```python
from build123d import *
from OCP.BRepFilletAPI import BRepFilletAPI_MakeChamfer

# Parameters (mm, degrees)
SKETCH_1_W                  = 85
SKETCH_1_H                  = 54
EXTRUDE_576_DEPTH           = 7.5
FILLET_627_R                = 3
CUT_EXTRUDE_1389_DEPTH      = 5.5
FILLET_1467_R               = 1
EXTRUDE_2395_DEPTH          = 2
CHAMFER_2448_SIZE           = 1
CHAMFER_2448_SIZE2          = 0.176326981
SKETCH_16_R                 = 2.5
CUT_EXTRUDE_2683_DEPTH      = 5
SKETCH_19_W                 = 7.62
SKETCH_19_H                 = 5.08
CUT_EXTRUDE_3124_DEPTH      = 10
SKETCH_21_W                 = 11.1
SKETCH_21_H                 = 1.1
CUT_EXTRUDE_2_DEPTH         = 10
SKETCH_22_W                 = 2.8
SKETCH_22_H                 = 1.2
CUT_EXTRUDE_3_DEPTH         = 10
CUT_EXTRUDE_5_DEPTH         = 10
SKETCH_30_W                 = 11.1
SKETCH_30_H                 = 0.725
SKETCH_30_W_2               = 2.8
SKETCH_30_H_2               = 1.3
CUT_EXTRUDE_6_DEPTH         = 1
EXTRUDE_2_DEPTH             = 1
EXTRUDE_3_DEPTH             = 1
CUT_EXTRUDE_START           = -1
SKETCH_31_W                 = 7.6
SKETCH_31_H                 = 0.55
SKETCH_31_W_2               = 5
SKETCH_31_H_2               = 2
CUT_EXTRUDE_7_DEPTH         = 1
SKETCH_32_W                 = 2.8
SKETCH_32_H                 = 1.2
CUT_EXTRUDE_8_DEPTH         = 10
SKETCH_33_W                 = 2.8
SKETCH_33_H                 = 1.3
CUT_EXTRUDE_9_DEPTH         = 2
SKETCH_34_R                 = 3
SKETCH_34_R_2               = 1.5
EXTRUDE_4_DEPTH             = 3.4
PATTERN_LINEAR_1_COUNT      = 2
PATTERN_LINEAR_1_PITCH      = 74
PATTERN_LINEAR_1_COUNT_DIR2 = 2
PATTERN_LINEAR_1_PITCH_DIR2 = 43


with BuildPart() as part:
    # 草图1 → Extrude 576 (new body)
    with BuildSketch(Plane(origin=(0, 0, 0), x_dir=(1, 0, 0), z_dir=(0, 1, 0))):
        Rectangle(SKETCH_1_W, SKETCH_1_H)
    extrude(amount=EXTRUDE_576_DEPTH)

    # Fillet 627
    fillet_627_edges = [part.edges().sort_by_distance(p)[0] for p in [
        (0, 0, 27),
        (-42.5, 0, 0),
        (0, 0, -27),
        (42.5, 0, 0),
        (42.5, 3.75, 27),
        (-42.5, 3.75, 27),
        (-42.5, 3.75, -27),
        (42.5, 3.75, -27),
    ]]
    fillet(fillet_627_edges, radius=FILLET_627_R)

    # 草图14 → Cut-Extrude 1389 (cut)
    with BuildSketch(Plane(origin=(0, 7.5, 0), x_dir=(1, 0, 0), z_dir=(0, 1, 0))):
        with BuildLine():
            Line((-39.5, -25), (39.5, -25))
            ThreePointArc((39.5, -25), (40.207106781, -24.707106781), (40.5, -24))
            Line((40.5, -24), (40.5, 24))
            ThreePointArc((40.5, 24), (40.207106781, 24.707106781), (39.5, 25))
            Line((39.5, 25), (-39.5, 25))
            ThreePointArc((-39.5, 25), (-40.207106781, 24.707106781), (-40.5, 24))
            Line((-40.5, 24), (-40.5, -24))
            ThreePointArc((-40.5, -24), (-40.207106781, -24.707106781), (-39.5, -25))
        make_face()
    extrude(amount=-CUT_EXTRUDE_1389_DEPTH, mode=Mode.SUBTRACT)

    # Fillet 1467
    fillet_1467_edges = [part.edges().sort_by_distance(p)[0] for p in [
        (40.207106781, 2, 24.707106781),
        (0, 2, 25),
        (-40.207106781, 2, 24.707106781),
        (-40.5, 2, 0),
        (-40.207106781, 2, -24.707106781),
        (0, 2, -25),
        (40.207106781, 2, -24.707106781),
        (40.5, 2, 0),
    ]]
    fillet(fillet_1467_edges, radius=FILLET_1467_R)

    # 草图15 → Extrude 2395 (add)
    with BuildSketch(Plane(origin=(0, 7.5, 0), x_dir=(1, 0, 0), z_dir=(0, 1, 0))):
        with BuildLine():
            Line((-39.5, -26), (39.5, -26))
            ThreePointArc((39.5, -26), (40.914213562, -25.414213562), (41.5, -24))
            Line((41.5, -24), (41.5, 24))
            ThreePointArc((41.5, 24), (40.914213562, 25.414213562), (39.5, 26))
            Line((39.5, 26), (-39.5, 26))
            ThreePointArc((-39.5, 26), (-40.914213562, 25.414213562), (-41.5, 24))
            Line((-41.5, 24), (-41.5, -24))
            ThreePointArc((-41.5, -24), (-40.914213562, -25.414213562), (-39.5, -26))
        make_face()
        with BuildLine():
            Line((-39.5, -25), (39.5, -25))
            ThreePointArc((39.5, -25), (40.207106781, -24.707106781), (40.5, -24))
            Line((40.5, -24), (40.5, 24))
            ThreePointArc((40.5, 24), (40.207106781, 24.707106781), (39.5, 25))
            Line((39.5, 25), (-39.5, 25))
            ThreePointArc((-39.5, 25), (-40.207106781, 24.707106781), (-40.5, 24))
            Line((-40.5, 24), (-40.5, -24))
            ThreePointArc((-40.5, -24), (-40.207106781, -24.707106781), (-39.5, -25))
        make_face(mode=Mode.SUBTRACT)
    extrude(amount=EXTRUDE_2395_DEPTH)

    # Chamfer 2448: one chamfer whose edges measure the first distance from different faces: ONE call of the kernel's chamfer builder (chamfer() names one face for all edges)
    chamfer_2448_edges_1 = [part.edges().sort_by_distance(p)[0] for p in [
        (-40.914213562, 9.5, 25.414213562),
    ]]
    chamfer_2448_side_1 = [part.faces().sort_by_distance(p)[0] for p in [
        (-40.914213562, 8.5, 25.414213562),
    ]]
    chamfer_2448_edges_2 = [part.edges().sort_by_distance(p)[0] for p in [
        (0, 9.5, 26),
    ]]
    chamfer_2448_side_2 = [part.faces().sort_by_distance(p)[0] for p in [
        (0, 8.5, 26),
    ]]
    chamfer_2448_edges_3 = [part.edges().sort_by_distance(p)[0] for p in [
        (40.914213562, 9.5, 25.414213562),
    ]]
    chamfer_2448_side_3 = [part.faces().sort_by_distance(p)[0] for p in [
        (40.914213562, 8.5, 25.414213562),
    ]]
    chamfer_2448_edges_4 = [part.edges().sort_by_distance(p)[0] for p in [
        (41.5, 9.5, 0),
    ]]
    chamfer_2448_side_4 = [part.faces().sort_by_distance(p)[0] for p in [
        (41.5, 8.5, 0),
    ]]
    chamfer_2448_edges_5 = [part.edges().sort_by_distance(p)[0] for p in [
        (40.914213562, 9.5, -25.414213562),
    ]]
    chamfer_2448_side_5 = [part.faces().sort_by_distance(p)[0] for p in [
        (40.914213562, 8.5, -25.414213562),
    ]]
    chamfer_2448_edges_6 = [part.edges().sort_by_distance(p)[0] for p in [
        (0, 9.5, -26),
    ]]
    chamfer_2448_side_6 = [part.faces().sort_by_distance(p)[0] for p in [
        (0, 8.5, -26),
    ]]
    chamfer_2448_edges_7 = [part.edges().sort_by_distance(p)[0] for p in [
        (-40.914213562, 9.5, -25.414213562),
    ]]
    chamfer_2448_side_7 = [part.faces().sort_by_distance(p)[0] for p in [
        (-40.914213562, 8.5, -25.414213562),
    ]]
    chamfer_2448_edges_8 = [part.edges().sort_by_distance(p)[0] for p in [
        (-41.5, 9.5, 0),
    ]]
    chamfer_2448_side_8 = [part.faces().sort_by_distance(p)[0] for p in [
        (-41.5, 8.5, 0),
    ]]
    chamfer_2448 = BRepFilletAPI_MakeChamfer(part.part.solid().wrapped)
    for e in chamfer_2448_edges_1:
        chamfer_2448.Add(CHAMFER_2448_SIZE, CHAMFER_2448_SIZE2, e.wrapped, chamfer_2448_side_1[0].wrapped)  # the first distance lies on this face
    for e in chamfer_2448_edges_2:
        chamfer_2448.Add(CHAMFER_2448_SIZE, CHAMFER_2448_SIZE2, e.wrapped, chamfer_2448_side_2[0].wrapped)  # the first distance lies on this face
    for e in chamfer_2448_edges_3:
        chamfer_2448.Add(CHAMFER_2448_SIZE, CHAMFER_2448_SIZE2, e.wrapped, chamfer_2448_side_3[0].wrapped)  # the first distance lies on this face
    for e in chamfer_2448_edges_4:
        chamfer_2448.Add(CHAMFER_2448_SIZE, CHAMFER_2448_SIZE2, e.wrapped, chamfer_2448_side_4[0].wrapped)  # the first distance lies on this face
    for e in chamfer_2448_edges_5:
        chamfer_2448.Add(CHAMFER_2448_SIZE, CHAMFER_2448_SIZE2, e.wrapped, chamfer_2448_side_5[0].wrapped)  # the first distance lies on this face
    for e in chamfer_2448_edges_6:
        chamfer_2448.Add(CHAMFER_2448_SIZE, CHAMFER_2448_SIZE2, e.wrapped, chamfer_2448_side_6[0].wrapped)  # the first distance lies on this face
    for e in chamfer_2448_edges_7:
        chamfer_2448.Add(CHAMFER_2448_SIZE, CHAMFER_2448_SIZE2, e.wrapped, chamfer_2448_side_7[0].wrapped)  # the first distance lies on this face
    for e in chamfer_2448_edges_8:
        chamfer_2448.Add(CHAMFER_2448_SIZE, CHAMFER_2448_SIZE2, e.wrapped, chamfer_2448_side_8[0].wrapped)  # the first distance lies on this face
    add(Compound.cast(chamfer_2448.Shape()), mode=Mode.REPLACE)

    # 草图16 → Cut-Extrude 2683 (cut)
    with BuildSketch(Plane(origin=(42.5, 0, 0), x_dir=(0, 0, -1), z_dir=(1, 0, 0))):
        with Locations((13, 7.5)):
            Circle(SKETCH_16_R)
    extrude(amount=-CUT_EXTRUDE_2683_DEPTH, mode=Mode.SUBTRACT)

    # 草图19 → Cut-Extrude 3124 (cut)
    with BuildSketch(Plane(origin=(42.5, 0, 0), x_dir=(0, 0, -1), z_dir=(1, 0, 0))):
        with Locations((-14.978380782, 7.5)):
            Rectangle(SKETCH_19_W, SKETCH_19_H)
    extrude(amount=-CUT_EXTRUDE_3124_DEPTH, mode=Mode.SUBTRACT)

    # 草图21 → 切除-拉伸2 (cut)
    with BuildSketch(Plane.ZY.offset(42.5)):
        with Locations((0, 8.225)):
            Rectangle(SKETCH_21_W, SKETCH_21_H)
    extrude(amount=-CUT_EXTRUDE_2_DEPTH, mode=Mode.SUBTRACT)

    # 草图22 → 切除-拉伸3 (cut)
    with BuildSketch(Plane.ZY.offset(42.5)):
        with Locations((15.5, 7.6)):
            Rectangle(SKETCH_22_W, SKETCH_22_H)
    extrude(amount=-CUT_EXTRUDE_3_DEPTH, mode=Mode.SUBTRACT)

    # 草图25 → 切除-拉伸5 (cut)
    with BuildSketch(Plane(origin=(42.5, 0, 0), x_dir=(0, 0, -1), z_dir=(1, 0, 0))):
        with BuildLine():
            Line((3.8, 8.257106781), (3.8, 8.95))
            ThreePointArc((3.8, 8.95), (3.653553391, 9.303553391), (3.3, 9.45))
            Line((3.3, 9.45), (-3.3, 9.45))
            ThreePointArc((-3.3, 9.45), (-3.653553391, 9.303553391), (-3.8, 8.95))
            Line((-3.8, 8.95), (-3.8, 8.257106781))
            ThreePointArc((-3.8, 8.257106781), (-3.761939766, 8.065765065), (-3.653553391, 7.903553391))
            Line((-3.653553391, 7.903553391), (-2.746446609, 6.996446609))
            ThreePointArc((-2.746446609, 6.996446609), (-2.584234935, 6.888060234), (-2.392893219, 6.85))
            Line((-2.392893219, 6.85), (2.392893219, 6.85))
            ThreePointArc((2.392893219, 6.85), (2.584234935, 6.888060234), (2.746446609, 6.996446609))
            Line((2.746446609, 6.996446609), (3.653553391, 7.903553391))
            ThreePointArc((3.653553391, 7.903553391), (3.761939766, 8.065765065), (3.8, 8.257106781))
        make_face()
    extrude(amount=-CUT_EXTRUDE_5_DEPTH, mode=Mode.SUBTRACT)

    # 草图30 → 切除-拉伸6 (cut)
    with BuildSketch(Plane.ZY.offset(41.5)):
        with Locations((0, 9.1375)):
            Rectangle(SKETCH_30_W, SKETCH_30_H)
        with Locations((15.5, 8.85)):
            Rectangle(SKETCH_30_W_2, SKETCH_30_H_2)
    extrude(amount=-CUT_EXTRUDE_6_DEPTH, mode=Mode.SUBTRACT)

    # 草图28 → 凸台-拉伸2 (add)
    with BuildSketch(Plane(origin=(41.5, 0, 0), x_dir=(0, 0, -1), z_dir=(1, 0, 0))):
        with BuildLine():
            Line((3.653553391, 7.903553391), (3.25, 7.5))
            Line((3.25, 7.5), (4.237115804, 7.5))
            Line((4.237115804, 7.5), (3.8, 8.257106781))
            ThreePointArc((3.8, 8.257106781), (3.761939766, 8.065765065), (3.653553391, 7.903553391))
        make_face()
        with BuildLine():
            Line((-3.25, 7.5), (-3.653553391, 7.903553391))
            ThreePointArc((-3.653553391, 7.903553391), (-3.761939766, 8.065765065), (-3.8, 8.257106781))
            Line((-3.8, 8.257106781), (-4.237115804, 7.5))
            Line((-4.237115804, 7.5), (-3.25, 7.5))
        make_face()
    extrude(amount=EXTRUDE_2_DEPTH)

    # 草图29 → 凸台-拉伸3 (add)
    with BuildSketch(Plane.ZY.offset(41.5)):
        Polygon((-5.55, 7.675), (-5.651036297, 7.5), (5.651036297, 7.5), (5.55, 7.675), align=None)
    extrude(amount=EXTRUDE_3_DEPTH)

    # 草图31 → 切除-拉伸7 (cut)
    with BuildSketch(Plane(origin=(41.5, 0, 0), x_dir=(0, 0, -1), z_dir=(1, 0, 0)).offset(CUT_EXTRUDE_START)):
        with Locations((0, 9.225)):
            Rectangle(SKETCH_31_W, SKETCH_31_H)
        with Locations((13, 8.5)):
            Rectangle(SKETCH_31_W_2, SKETCH_31_H_2)
    extrude(amount=CUT_EXTRUDE_7_DEPTH, mode=Mode.SUBTRACT)

    # 草图32 → 切除-拉伸8 (cut)
    with BuildSketch(Plane(origin=(0, 0, -27), x_dir=(-1, 0, 0), z_dir=(0, 0, -1))):
        with Locations((31, 7.6)):
            Rectangle(SKETCH_32_W, SKETCH_32_H)
    extrude(amount=-CUT_EXTRUDE_8_DEPTH, mode=Mode.SUBTRACT)

    # 草图33 → 切除-拉伸9 (cut)
    with BuildSketch(Plane(origin=(0, 0, -27), x_dir=(-1, 0, 0), z_dir=(0, 0, -1))):
        with Locations((31, 8.85)):
            Rectangle(SKETCH_33_W, SKETCH_33_H)
    extrude(amount=-CUT_EXTRUDE_9_DEPTH, mode=Mode.SUBTRACT)

    # 草图34 → 凸台-拉伸4 (add)
    with BuildSketch(Plane(origin=(0, 2, 0), x_dir=(1, 0, 0), z_dir=(0, 1, 0))):
        with Locations(Location((-37, 21.5, 0), (0, 0, 123.557309761))):
            Circle(SKETCH_34_R)
        with Locations(Location((-37, 21.5, 0), (0, 0, 270))):
            Circle(SKETCH_34_R_2, mode=Mode.SUBTRACT)
    extrude_4 = extrude(amount=EXTRUDE_4_DEPTH)

    # 阵列(线性)1: Extrude 4 2 × 2
    with Locations(*[(i * PATTERN_LINEAR_1_PITCH, 0, j * PATTERN_LINEAR_1_PITCH_DIR2) for i in range(PATTERN_LINEAR_1_COUNT) for j in range(PATTERN_LINEAR_1_COUNT_DIR2) if (i, j) != (0, 0)]):
        add(extrude_4)


solid = part.part
```
Read the model definition and answer for the solid it produces. Units are mm, in the model's axes. A direction names the side the tool comes from. Coordinates: 2 decimals unless noted, no trailing zeros. Order: outer loops, then holes, each group sorted by start corner. A loop starts at its lowest first (then second) coordinate and runs counter-clockwise, first axis right, second up. Notation, with made-up numbers: (-10, 72) - (28, 72) arc R27 cw to (28, 104) - close; hole circle Ø10 at (51.25, 75). An arc over 180 degrees is marked (long way). Answer as a JSON object with one key per item and string values. Group by question number.
Item 1: Section C-C (x = -31) is taken. Give the vertices of the cut face in (y, z), plus the area to 3 significant figures.
Item 2: Section B-B (z = -13) is taken. Give the vertices of the cut face in (x, y).
Item 3: Flat-ended cylindrical pins translate along their axes: P1, Ø4, axis at x = -37, z = -21.5, coming from the +Y side; P2, Ø2, axis at y = 8, z = -26.5, coming from the +X side; P3, Ø1.6, axis at x = 41.5, y = 8, coming from the -Z side. Find the tip coordinate at first contact, or state that the pin passes through.
Item 4: The mould has two halves that part along Z. Classify faces 5 (the face through (37, 2, 21)), 6 (the face through (40.9, 9, -25.3)), 7 (the face through (-41.64, 0.9, -0.34)): +Z half, -Z half, draft (parallel to the pull), parting line (faces both ways), or undercut.
Item 5: Consider probe 1 along X at (y, z) = (4.6, -21.5); probe 2 along Z at (x, y) = (12.5, 8.5); probe 3 along Z at (x, y) = (22, 3). Determine where each line is inside the solid, lowest interval first. Write a range as from..to.
Item 6: Section A-A (x = 9) is taken. Give the vertices of the cut face in (y, z), plus the area to 3 significant figures.
Item 7: A tool of negligible diameter and unlimited length cuts with its end or side. For faces 1 (the face through (40.93, 7.99, -25.4)), 2 (the face through (-40.93, 7.99, 25.4)), 3 (the face through (-1, 6, 25)), 4 (the face through (41, 7, 18.788)), from which of +Z, -Z, +X, -X, +Y, -Y can it reach the whole face along a straight path? Write none if from no direction.
Results are:
{
 "1": {"outline": "(0, -24) arc R3 ccw to (3, -27) - (7, -27) - (7, -25) - (3, -25) arc R1 cw to (2, -24) - (2, 24) arc R1 cw to (3, 25) - (9.5, 25) - (9.5, 25.82) - (8.5, 26) - (7.5, 26) - (7.5, 27) - (3, 27) arc R3 ccw to (0, 24) - close", "area": "127 mm^2"},
 "2": {"outline": "(-42.5, 3) arc R3 ccw to (-39.5, 0) - (39.5, 0) arc R3 ccw to (42.5, 3) - (42.5, 5) - (40.5, 5) - (40.5, 3) arc R1 cw to (39.5, 2) - (-39.5, 2) arc R1 cw to (-40.5, 3) - (-40.5, 9.5) - (-41.32, 9.5) - (-41.5, 8.5) - (-41.5, 7.5) - (-42.5, 7.5) - close"},
 "3": {"P1": "stops at y = 5.4", "P2": "stops at x = 42.02", "P3": "stops at z = -26.67"},
 "4": {"face 5": "undercut", "face 6": "-Z half", "face 7": "draft"},
 "5": {"probe 1": "x = -42.5..-40.5, -40..-38.5, -35.5..-34, 34..35.5, 38.5..40, 40.5..42.5", "probe 2": "z = -26..-25, 25..26", "probe 3": "z = -27..-25, 25..27"},
 "6": {"outline": "(0, -24) arc R3 ccw to (3, -27) - (7.5, -27) - (7.5, -26) - (8.5, -26) - (9.5, -25.82) - (9.5, -25) - (3, -25) arc R1 cw to (2, -24) - (2, 24) arc R1 cw to (3, 25) - (9.5, 25) - (9.5, 25.82) - (8.5, 26) - (7.5, 26) - (7.5, 27) - (3, 27) arc R3 ccw to (0, 24) - close", "area": "130 mm^2"},
 "7": {"face 1": "-Z, +X, +Y", "face 2": "+Z, -X, +Y", "face 3": "+Y", "face 4": "+X, +Y"}
}
